from build123d import *

# Parameters (mm, degrees)
SKETCH1_W           = 8
SKETCH1_H           = 12
BOSS_EXTRUDE1_DEPTH = 10
SKETCH2_R           = 2.5
BOSS_EXTRUDE2_DEPTH = 10
FILLET1_R           = 1
FILLET2_R           = 1


with BuildPart() as part:
    # Sketch1 → Boss-Extrude1 (new body)
    with BuildSketch(Plane(origin=(0, 0, 0), x_dir=(1, 0, 0), z_dir=(0, 1, 0))):
        with Locations((4, 6)):
            Rectangle(SKETCH1_W, SKETCH1_H)
    extrude(amount=BOSS_EXTRUDE1_DEPTH)

    # Sketch2 → Boss-Extrude2 (add)
    with BuildSketch(Plane(origin=(0, 10, 0), x_dir=(1, 0, 0), z_dir=(0, 1, 0))):
        with Locations(Location((4, 6, 0), (0, 0, 270))):
            Circle(SKETCH2_R)
    extrude(amount=BOSS_EXTRUDE2_DEPTH)

    # Fillet1
    fillet1_edges = [part.edges().sort_by_distance(p)[0] for p in [
        (4, 20, -8.5),
    ]]
    fillet(fillet1_edges, radius=FILLET1_R)

    # Fillet2
    fillet2_edges = [part.edges().sort_by_distance(p)[0] for p in [
        (0, 5, -12),
        (8, 5, -12),
        (8, 5, 0),
        (0, 5, 0),
    ]]
    fillet(fillet2_edges, radius=FILLET2_R)


solid = part.part
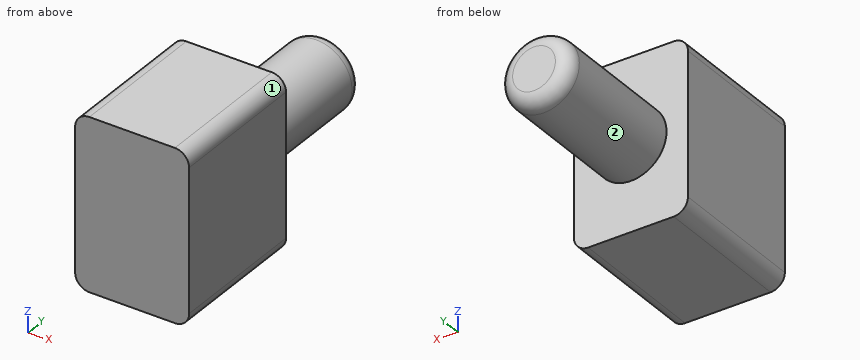
CAD build for the part. Positions are in the model's coordinates, mm. Face numbers are marked on the shaded views. A direction names the side the tool comes from. Round coordinates to 2 decimals unless told otherwise and drop trailing zeros. Write each loop counter-clockwise with the first axis right and the second up, starting at its lowest first coordinate (ties: lowest second). Pieces come first, ordered by that corner, then holes.
(1) Slice it at C-C, the plane y = 14.5. Write the cut outline in (x, z).
(2) 3-axis set-ups, long thin cutter, end or side, ignore diameter. For the marked faces 1 and 2: which of +Z, -Z, +X, -X, +Y, -Y reach the whole face in a straight line?
(3) Slice it at A-A, the plane z = -6. Write the cut outline in (x, y), and give its area (3 significant figures).
(4) Slice it at B-B, the plane x = 4. Write the cut outline in (y, z).
(5) Drop flat-ended pins along their axis: P1, Ø1, axis at x = 3, z = -2.5, coming from the +Y side; P2, Ø1, axis at x = 4, y = 18, coming from the -Z side. Give the stop position or say it passes through.
(6) Probe line 1 along Y through (x, z) = (6.75, -6.5); line 2 along X through (y, z) = (12.75, -6); line 3 along X through (y, z) = (15.25, -3.75). List the from-to ranges inside material, lowest first.
(7) Slice it at D-D, the plane x = 1.25. Write the cut outline in (y, z).
From the geometry:
1. outline: circle Ø5 at (4, -6)
2. face 1: +Z, +X, +Y, -Y
2. face 2: +Y
3. outline: (0, 0) - (8, 0) - (8, 10) - (6.5, 10) - (6.5, 19) arc R1 ccw to (5.5, 20) - (2.5, 20) arc R1 ccw to (1.5, 19) - (1.5, 10) - (0, 10) - close
3. area: 130 mm2
4. outline: (0, -12) - (10, -12) - (10, -8.5) - (19, -8.5) arc R1 ccw to (20, -7.5) - (20, -4.5) arc R1 ccw to (19, -3.5) - (10, -3.5) - (10, 0) - (0, 0) - close
5. P1: stops at y = 10
5. P2: stops at z = -8.5
6. line 1: y = 0 to 10
6. line 2: x = 1.5 to 6.5
6. line 3: x = 2.91 to 5.09
7. outline: (0, -12) - (10, -12) - (10, 0) - (0, 0) - close
